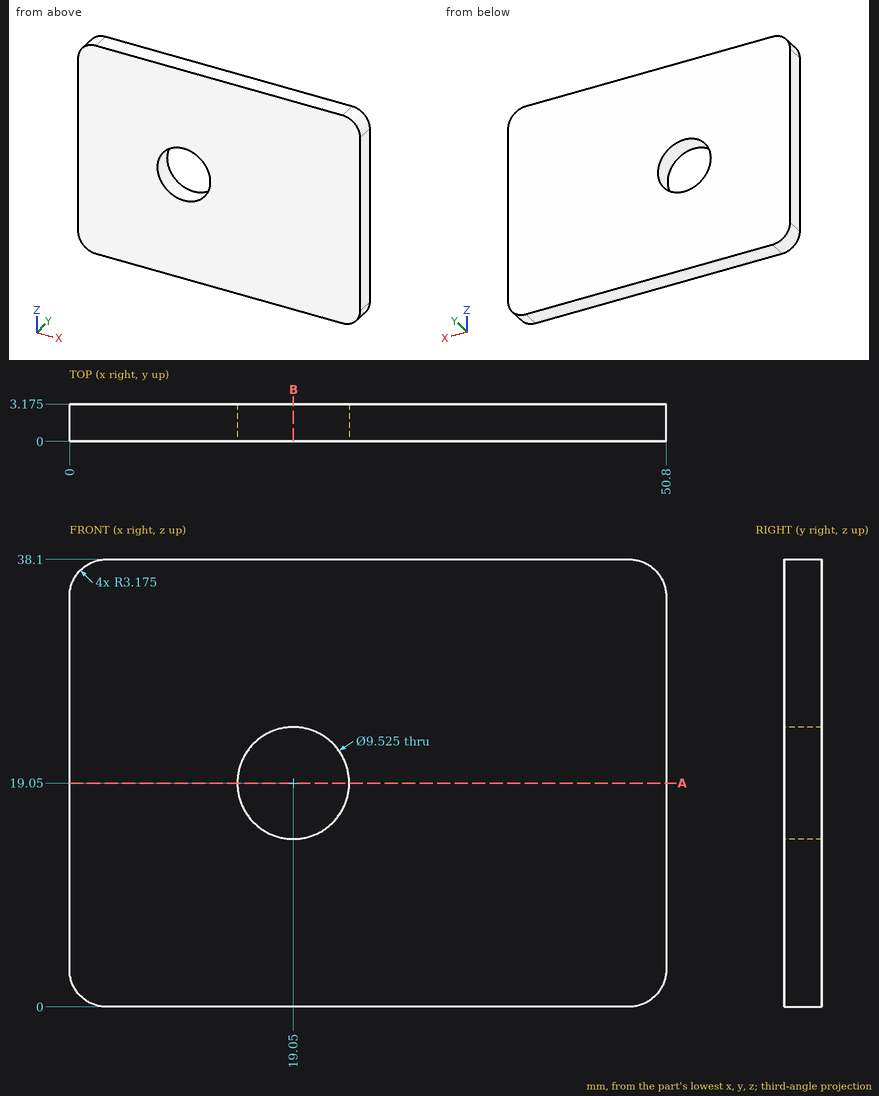
Drawing for the job (mm, zero at the part's lowest x, y, z). Round coordinates to 2 decimals unless told otherwise and drop trailing zeros. Write each loop counter-clockwise with the first axis right and the second up, starting at its lowest first coordinate (ties: lowest second). Pieces come first, ordered by that corner, then holes. Notation, with made-up numbers: (-3, 35.5) - (30, 35.5) arc R15 ccw to (30, 43.5) - close; hole circle Ø4 at (63, 2.25). An arc over 180 degrees is marked (long way). Use CSV: the item, a comma, the result in double quotes.
(1) Pin check, flat tip, straight feed: P1, Ø12.5, axis at x = 19.05, z = 19.05, coming from the +Y side (3 decimals). Stop position of the tip, or through.
Response:
P1,"y = 3.175"
(2) Wall check: line 1 (X direction, y = 1.05, z = 19.05); line 2 (Z direction, x = 19.05, y = 1.9); line 3 (X direction, y = 0.95, z = 20). Give the ranges that are in metal, low to high.
Response:
line 1,"0 to 14.29, 23.81 to 50.8"
line 2,"0 to 14.29, 23.81 to 38.1"
line 3,"0 to 14.38, 23.72 to 50.8"
(3) Band-saw the part on A-A (z = 19.05). Write the cut outline in (x, y) (1 decimal), plus the area to 3 significant figures.
Response:
outline,"(0, 0) - (14.3, 0) - (14.3, 3.2) - (0, 3.2) - close; (23.8, 0) - (50.8, 0) - (50.8, 3.2) - (23.8, 3.2) - close"
area,"131 mm²"
(4) Band-saw the part on B-B (x = 19.05). Write the cut outline in (y, z) (1 decimal).
Response:
outline,"(0, 0) - (3.2, 0) - (3.2, 14.3) - (0, 14.3) - close; (0, 23.8) - (3.2, 23.8) - (3.2, 38.1) - (0, 38.1) - close"
